For this review, take the finished solid that the model builds, in its own axes (mm). Face numbers are marked on the shaded views. A direction names the side the tool comes from. Give positions to 0.01 mm unless a question says otherwise; leave off trailing zeros. Write each loop counter-clockwise with the first axis right and the second up, starting at its lowest first coordinate (ties: lowest second). Pieces come first, ordered by that corner, then holes. Notation, with made-up numbers: (88, 44.25) -> (131, 44.25) arc R31 ccw to (131, 71.25) -> close; hole circle Ø5 at (-25.5, 46). An arc over 180 degrees is marked (long way). Write item = value, one per line.
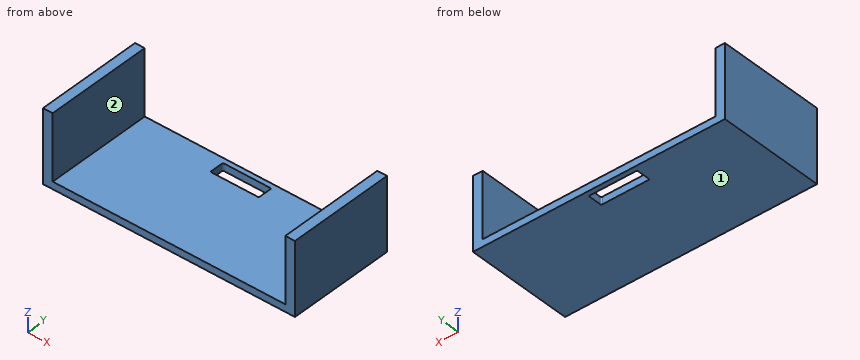
```python
from build123d import *

# Parameters (mm, degrees)
F0_W     = 1320.8
F0_H     = 558.8
F1_DEPTH = 38.1
F2_W     = 254
F2_H     = 76.2
F3_DEPTH = 333.248
F4_R     = 6.35
F5_DEPTH = 342.9


with BuildPart() as f1:
    # F0 (on Top) → F1 (new body)
    with BuildSketch(Plane.XY):
        with Locations((0.0168122351, -382.5642513233)):
            Rectangle(F0_W, F0_H)
    extrude(amount=F1_DEPTH)

    # F2 (on face) → F3 (cut, symmetric)
    with BuildSketch(Plane.XY.offset(38.1)):
        with Locations((-50.7831877649, -166.6642513233)):
            Rectangle(F2_W, F2_H)
    extrude(amount=F3_DEPTH, both=True, mode=Mode.SUBTRACT)

    # F4
    f4_edges = [f1.edges().sort_by_distance(p)[0] for p in [
        (-177.783188, -128.564251, 19.05),
        (-177.783188, -204.764251, 19.05),
        (76.216812, -128.564251, 19.05),
        (76.216812, -204.764251, 19.05),
    ]]
    fillet(f4_edges, radius=F4_R)

    # F2 (on face) → F5 (join)
    with BuildSketch(Plane.XY.offset(38.1)):
        Polygon((-609.5831877649, -103.1642513233), (-660.3831877649, -103.1642513233), (-660.3831877649, -661.9642513233), (-609.5831877649, -661.9642513233), (-609.5831877649, -319.0642513233), (-609.5831877649, -300.0142513233), align=None)
        Polygon((660.4168122351, -103.1642513233), (609.6168122351, -103.1642513233), (609.6168122351, -300.0142513233), (609.6168122351, -319.0642513233), (609.6168122351, -661.9642513233), (660.4168122351, -661.9642513233), align=None)
    extrude(amount=F5_DEPTH)


solid = f1.part
```
(1) Take a section at D-D (x = 381.5). Write out the cut boundary in (y, z), plus the area to 3 significant figures.
Answers below:
outline = (-661.96, 0) -> (-103.16, 0) -> (-103.16, 38.1) -> (-661.96, 38.1) -> close
area = 21,300 mm^2
(2) Take a section at A-A (z = 332.5). Write out the cut boundary in (x, y).
Answers below:
outline = (-660.38, -661.96) -> (-609.58, -661.96) -> (-609.58, -103.16) -> (-660.38, -103.16) -> close; (609.62, -661.96) -> (660.42, -661.96) -> (660.42, -103.16) -> (609.62, -103.16) -> close
(3) Take a section at B-B (y = -150.5). Write out the cut boundary in (x, z), plus the area to 3 significant figures.
Answers below:
outline = (-660.38, 0) -> (-177.78, 0) -> (-177.78, 38.1) -> (-609.58, 38.1) -> (-609.58, 381) -> (-660.38, 381) -> close; (76.22, 0) -> (660.42, 0) -> (660.42, 381) -> (609.62, 381) -> (609.62, 38.1) -> (76.22, 38.1) -> close
area = 75,500 mm^2
(4) To check wall thickness, follow probe 1 along X at (y, z) = (-540, 85); probe 2 along Z at (x, y) = (-585, -465.5). State the ranges of each line that lie inside material, in increasing order.
Answers below:
probe_1 = -660.38 to -609.58, 609.62 to 660.42
probe_2 = 0 to 38.1
(5) Tool access review of the marked faces 1 and 2: name each direction out of +Z, -Z, +X, -X, +Y, -Y from which nothing blocks a thin tool from reaching the whole face with its end or side.
Answers below:
face_1 = -Z, +X, -X, +Y, -Y
face_2 = +Z, +Y, -Y
(6) For pin 1 (5 mm diameter, centred on x = -257.5, y = -272, fed in from +Z), flat-tipped, find the tip position at first contact; note if it passes through.
Answers below:
pin_1 = 38.1
(7) Take a section at C-C (y = -607.5). Write out the cut boundary in (x, z).
Answers below:
outline = (-660.38, 0) -> (660.42, 0) -> (660.42, 381) -> (609.62, 381) -> (609.62, 38.1) -> (-609.58, 38.1) -> (-609.58, 381) -> (-660.38, 381) -> close
